Check sheet for the modelled part. Datum: model origin and axes. Units: mm. A direction names the side the tool comes from. Round coordinates to 2 decimals unless told otherwise and drop trailing zeros. Loops run counter-clockwise (first coordinate to the right, second up) from the corner with the lowest first, then second, coordinate; pieces in that order, holes last. Notation, with made-up numbers: (-7.5, 39) -> (23.5, 39) arc R27 ccw to (23.5, 78) -> close; hole circle Ø1 at (-0.75, 23). An arc over 180 degrees is marked (long way). One line per item, written item: value. Start each with the question number.
1. Release check for a two-part mould opening along X. For faces 1 (the face through (-18.807, 16.868, -24.395)), 2 (the face through (-25.133, 1.375, 32.567)), 3 (the face through (1, -9, 1)), 4 (the face through (50.5, -7, 9)) record: +X half, -X half, draft (parallel to the pull), parting line (faces both ways), or undercut.
2. Cross-section at A-A on x = 40.5. Record the cut outline in (y, z).
3. Cross-section at B-B on z = -23.5. Record the cut outline in (x, y), then the cut area to 3 significant figures.
4. Cross-section at C-C on y = 0.75. Record the cut outline in (x, z).
5. Go/stop test with flat-tipped pins: pin 1 (6.5 mm diameter, centred on y = 5, z = -3.5, fed in from +X); pin 2 (1 mm diameter, centred on y = -3.5, z = 30, fed in from +X). Record where each tip stops, or that it passes through.
6. Cross-section at D-D on z = 13.5. Record the cut outline in (x, y).
7. Set-up check for faces 5 (the face through (1, 4, -31.5)), 6 (the face through (-37.24, 16.87, -24.54)), 7 (the face through (-38.59, 1.49, 32.57)), 8 (the face through (-1, -2, 30)): record each of +Z, -Z, +X, -X, +Y, -Y from which the full face is reachable in a straight line by a thin tool's end or side.
8. Material ranges on L1, parallel to Z at x = 4.5, y = 7.75; L2, parallel to Y at x = -25, z = -2.5; L3, parallel to Z at x = 3.5, y = -2.75, recorded low to high.
from build123d import *

# Parameters (mm, degrees)
SKETCH003_W      = 27.1
SKETCH003_H      = 65.3
EXTRUDE002_DEPTH = 2.5
SKETCH004_W      = 2
SKETCH004_H      = 2
PAD003_DEPTH     = 90
SKETCH005_W      = 27.1
SKETCH005_H      = 65.3
SKETCH005_W_2    = 22.1
SKETCH005_H_2    = 60.3
PAD004_DEPTH     = 96
POCKET_DEPTH     = 2.5
POCKET001_DEPTH  = 2.5
FILLET_R         = 1


with BuildPart() as part:
    # Sketch003 → Extrude002 (new body)
    with BuildSketch(Plane(origin=(-45.5, -6.5, -29), x_dir=(0, -1, 0), z_dir=(-1, 0, 0))):
        with Locations((-11.05, 30.15)):
            Rectangle(SKETCH003_W, SKETCH003_H)
    extrude(amount=EXTRUDE002_DEPTH)

    # Sketch004 → Pad003 (new body)
    with BuildSketch(Plane.YZ.offset(-45.5)):
        with Locations((-3, -28)):
            Rectangle(SKETCH004_W, SKETCH004_H)
        with Locations((-3, 30.3)):
            Rectangle(SKETCH004_W, SKETCH004_H)
    extrude(amount=PAD003_DEPTH)

    # Sketch005 → Pad004 (new body)
    with BuildSketch(Plane.YZ.offset(-45.5)):
        with Locations((4.55, 1.15)):
            Rectangle(SKETCH005_W, SKETCH005_H)
        with Locations((4.55, 1.15)):
            Rectangle(SKETCH005_W_2, SKETCH005_H_2, mode=Mode.SUBTRACT)
    extrude(amount=PAD004_DEPTH)

    # Sketch006 → Pocket (cut)
    with BuildSketch(Plane.XY.offset(33.8)):
        with BuildLine():
            ThreePointArc((-35.90548, 4.1175), (-38.58891, 1.43407), (-35.90548, -1.24936))
            Line((-35.90548, -1.24936), (-27.8154, -1.24936))
            ThreePointArc((-27.8154, -1.24936), (-25.13197, 1.43407), (-27.8154, 4.1175))
            Line((-35.90548, 4.1175), (-27.8154, 4.1175))
        make_face()
    extrude(amount=-POCKET_DEPTH, mode=Mode.SUBTRACT)

    # Sketch007 → Pocket001 (cut)
    with BuildSketch(Plane(origin=(0, 18.1, 0), x_dir=(-1, 0, 0), z_dir=(0, 1, 0))):
        with BuildLine():
            ThreePointArc((22.1471, -21.12672), (18.8058, -24.46802), (22.1471, -27.80932))
            Line((22.1471, -27.80932), (33.8994, -27.80932))
            ThreePointArc((33.8994, -27.80932), (37.2407, -24.46802), (33.8994, -21.12672))
            Line((22.1471, -21.12672), (33.8994, -21.12672))
        make_face()
    extrude(amount=-POCKET001_DEPTH, mode=Mode.SUBTRACT)

    # Fillet
    fillet_edges = [part.edges().sort_by_distance(p)[0] for p in [
        (2.5, -9, 33.8),
        (2.5, -9, -31.5),
        (-46.75, -9, -31.5),
        (-46.75, -9, 33.8),
        (-48, -9, 1.15),
        (-48, 4.55, 33.8),
        (-48, 18.1, 1.15),
        (-48, 4.55, -31.5),
        (2.5, 18.1, 33.8),
        (-46.75, 18.1, 33.8),
        (-46.75, 18.1, -31.5),
        (2.5, 18.1, -31.5),
    ]]
    fillet(fillet_edges, radius=FILLET_R)


solid = part.part
Taken from the geometry:
1. face 1: undercut
1. face 2: undercut
1. face 3: draft
1. face 4: +X half
2. outline: (-9, -30.5) arc R1 ccw to (-8, -31.5) -> (17.1, -31.5) arc R1 ccw to (18.1, -30.5) -> (18.1, 32.8) arc R1 ccw to (17.1, 33.8) -> (-8, 33.8) arc R1 ccw to (-9, 32.8) -> close; hole (-6.5, -29) -> (-4, -29) -> (-4, -27) -> (-2, -27) -> (-2, -29) -> (15.6, -29) -> (15.6, 31.3) -> (-2, 31.3) -> (-2, 29.3) -> (-4, 29.3) -> (-4, 31.3) -> (-6.5, 31.3) -> close
3. outline: (-48, -8) arc R1 ccw to (-47, -9) -> (50.5, -9) -> (50.5, -6.5) -> (-45.5, -6.5) -> (-45.5, 15.6) -> (-37.1, 15.6) -> (-37.1, 18.1) -> (-47, 18.1) arc R1 ccw to (-48, 17.1) -> close; (-18.95, 15.6) -> (50.5, 15.6) -> (50.5, 18.1) -> (-18.95, 18.1) -> close
3. area: 502 mm2
4. outline: (-48, -30.5) arc R1 ccw to (-47, -31.5) -> (50.5, -31.5) -> (50.5, -29) -> (-45.5, -29) -> (-45.5, 31.3) -> (-38.5, 31.3) -> (-38.5, 33.8) -> (-47, 33.8) arc R1 ccw to (-48, 32.8) -> close; (-25.22, 31.3) -> (50.5, 31.3) -> (50.5, 33.8) -> (-25.22, 33.8) -> close
5. pin 1: stops at x = -45.5
5. pin 2: stops at x = 44.5
6. outline: (-48, -8) arc R1 ccw to (-47, -9) -> (50.5, -9) -> (50.5, -6.5) -> (-45.5, -6.5) -> (-45.5, 15.6) -> (50.5, 15.6) -> (50.5, 18.1) -> (-47, 18.1) arc R1 ccw to (-48, 17.1) -> close
7. face 5: -Z, +X, -X, +Y, -Y
7. face 6: +Y
7. face 7: +Z
7. face 8: +X
8. L1: z = -31.5 to -29, 31.3 to 33.8
8. L2: y = -9 to -6.5, 15.6 to 18.1
8. L3: z = -31.5 to -27, 29.3 to 33.8
